from build123d import *

# Parameters (mm, degrees)
SKETCH1_R           = 35
BOSS_EXTRUDE1_DEPTH = 2
SKETCH3_R           = 9.9
BOSS_EXTRUDE2_DEPTH = 3


with BuildPart() as part:
    # Sketch1 → Boss-Extrude1 (new body)
    with BuildSketch(Plane(origin=(0, 0, 0), x_dir=(1, 0, 0), z_dir=(0, 1, 0))):
        Circle(SKETCH1_R)
    extrude(amount=BOSS_EXTRUDE1_DEPTH)

    # Sketch3 → Boss-Extrude2 (add)
    with BuildSketch(Plane.XZ):
        with Locations((25.1, 0)):
            Circle(SKETCH3_R)
        with Locations((0, -25.1)):
            Circle(SKETCH3_R)
        with Locations((-25.1, 0)):
            Circle(SKETCH3_R)
        with Locations((0, 25.1)):
            Circle(SKETCH3_R)
    extrude(amount=BOSS_EXTRUDE2_DEPTH)


solid = part.part
CAD build for the part. Positions are in the model's coordinates, mm. A direction names the side the tool comes from. Round coordinates to 2 decimals unless told otherwise and drop trailing zeros. Write each loop counter-clockwise with the first axis right and the second up, starting at its lowest first coordinate (ties: lowest second). Pieces come first, ordered by that corner, then holes.
(1) Drop flat-ended pins along their axis: P1, Ø3, axis at y = -1, z = -21.5, coming from the -X side; P2, Ø1, axis at x = 6.5, y = -1.5, coming from the +Z side; P3, Ø1.5, axis at x = -7.5, y = -0.5, coming from the +Z side. Give the stop position or say it passes through.
(2) 3-axis set-ups, long thin cutter, end or side, ignore diameter. For faces 4 (the face through (-2.146, -1.479, 15.435)), 5 (the face through (0, -3, 25)): which of +Z, -Z, +X, -X, +Y, -Y reach the whole face in a straight line?
(3) Slice it at C-C, the plane y = 0.8. Write the cut outline in (x, z), and give its area (3 significant figures).
(4) Slice it at A-A, the plane x = 25.1. Write the cut outline in (y, z).
(5) Mould opens along Z. For faces 1 (the face through (-35, -1, 0)), 2 (the face through (-25, -3, 0)), 3 (the face through (0, 0, 0)) say: pulls with the +Z half, pulls with the -Z half, needs draft (parallel to the pull), parting line crosses it, or undercut.
(6) Slice it at B-B, the plane z = 17. Write the cut outline in (x, y), and give its area (3 significant figures).
(7) Probe line 1 along X through (y, z) = (-1.2, 0.5); line 2 along Y through (x, z) = (-22.5, 14.5); line 3 along X through (y, z) = (-0.5, 2). List the from-to ranges inside material, lowest first.
From the geometry:
1. P1: stops at x = -28.45
1. P2: stops at z = 32.97
1. P3: stops at z = 34.3
2. face 4: -Y
2. face 5: +Z, -Z, +X, -X, -Y
3. outline: circle Ø70 at (0, 0)
3. area: 3,850 mm2
4. outline: (-3, -9.9) - (0, -9.9) - (0, -24.39) - (2, -24.39) - (2, 24.39) - (0, 24.39) - (0, 9.9) - (-3, 9.9) - close
5. face 1: parting line crosses it
5. face 2: needs draft
5. face 3: undercut
6. outline: (-30.59, 0) - (-5.69, 0) - (-5.69, -3) - (5.69, -3) - (5.69, 0) - (30.59, 0) - (30.59, 2) - (-30.59, 2) - close
6. area: 157 mm2
7. line 1: x = -34.99 to -15.21, 15.21 to 34.99
7. line 2: y = 0 to 2
7. line 3: x = -34.8 to -15.4, 15.4 to 34.8
